Read the model definition and answer for the solid it produces. Units are mm, in the model's axes. A direction names the side the tool comes from. Coordinates: 2 decimals unless noted, no trailing zeros. Write each loop counter-clockwise with the first axis right and the second up, starting at its lowest first coordinate (ties: lowest second). Pieces come first, ordered by that corner, then holes.
(1) Find the intervals of material crossed by probe 1 along Y at (x, z) = (-76, -3); probe 2 along Z at (x, y) = (-47, -22); probe 3 along Z at (x, y) = (-68, -23.5), in increasing order.
(2) Given pin 1 (1 mm diameter, centred on x = -35, y = -8.5, fed in from +Z); pin 2 (6 mm diameter, centred on x = -29, z = -38, fed in from +Y); pin 3 (8 mm diameter, centred on x = -19, y = -14, fed in from +Z); pin 4 (4 mm diameter, centred on x = -33.5, y = -19.5, fed in from -Z), each flat-ended and moving along its own axis, determine where each tip first touches the part or whether it passes through.
(3) The mould has two halves that part along Z. Classify faces 1 (the cylindrical face through (-58.34, -3.22, 16.94)), 2 (the cylindrical face through (-85.704, -15.653, -1.885)), 3 (the flat face through (-33, 0, 1)): +Z half, -Z half, draft (parallel to the pull), parting line (faces both ways), or undercut.
(4) Section A-A on x = -27.5 is taken. Write down the section's boundary in (y, z), then the cut area to 3 significant figures.
(5) Which of the six approach directions +Z, -Z, +X, -X, +Y, -Y give full straight-line access (tool end or side, diameter ignored) to faces 4 (the flat face through (-31, -6.35, 1)), 5 (the cylindrical face through (-36.031, -3.219, -48.252))?
(6) Section D-D on x = -7.5 is taken. Write down the section's boundary in (y, z), then the cut area to 3 significant figures.
Autodesk Inventor part; units mm, degrees
ref_plane "YZ Plane" through (0, 0, 0) normal (1, 0, 0) x (0, 1, 0)
ref_plane "XZ Plane" through (0, 0, 0) normal (0, 1, 0) x (-1, 0, 0)
ref_plane "XY Plane" through (0, 0, 0) normal (0, 0, 1) x (1, 0, 0)
sketch "Sketch1" plane through (0, 0, 0) normal (0, 1, 0) x (-1, 0, 0)
  circle A0 centre (0, 0) radius 85.725
  dimension "d0" = 171.45
extrude "Extrusion1" add sketch "Sketch1" against normal blind 6.35
sketch "Sketch2" plane through (0, -6.35, 0) normal (0, -1, 0) x (1, 0, 0)
  circle A0 centre (0, 0) radius 85.725
  circle A1 centre (0, 0) radius 80.9625
  dimension "d3" = 161.925
extrude "Extrusion2" add sketch "Sketch2" along normal blind 25.4
sketch "Sketch3" plane through (0, 0, 0) normal (0, 1, 0) x (1, 0, 0)
  arc A0 (0, -85.725) -> (0, 85.725) centre (0, 0) ccw
  circle A1 centre (0, 0) radius 85.725
  line L0 (0, 85.725) -> (0, -85.725)
extrude "Extrusion3" cut sketch "Sketch3" against normal through all contours L0 A0
sketch "Sketch4" plane through (0, 0, 0) normal (0, 1, 0) x (1, 0, 0)
  circle A0 centre (0, 0) radius 63.5 construction
  line L0 (0, 0) -> (-37.3244, -51.3726) construction
  line L1 (0, -85.725) -> (0, 85.725) construction
  point P0 (-60.3921, -19.6226)
  point P1 (-60.3921, 19.6226)
  point P2 (-37.3244, 51.3726)
  point P3 (0, 63.5)
  point P4 (37.3244, 51.3726)
  point P5 (60.3921, 19.6226)
  point P6 (60.3921, -19.6226)
  point P7 (37.3244, -51.3726)
  point P8 (0, -63.5)
  dimension "d8" = 127
  dimension "d9" = 36
  dimension "d12" = 360
hole "Hole1" at (-37.3244, 0, 51.3726) at (-60.3921, 0, 19.6226) at (-60.3921, 0, -19.6226) at (-37.3244, 0, -51.3726) at (0, 0, -63.5) at (37.3244, 0, -51.3726) at (60.3921, 0, -19.6226) at (60.3921, 0, 19.6226) at (37.3244, 0, 51.3726) at (0, 0, 63.5) direction (0, -1, 0) diameter 6.7564 end through all
properties part number "CoverPlateForWaterHalf" material "PET Plastic"
Response:
1. probe 1: y = -6.35 to 0
1. probe 2: z = -71.69 to -65.92, 65.92 to 71.69
1. probe 3: z = -52.2 to -43.94, 43.94 to 52.2
2. pin 1: stops at z = 78.48
2. pin 2: stops at y = 0
2. pin 3: stops at z = 84.4
2. pin 4: stops at z = -79.73
3. face 1: undercut
3. face 2: parting line
3. face 3: draft
4. outline: (-31.75, -81.19) - (0, -81.19) - (0, 81.19) - (-31.75, 81.19) - (-31.75, 76.15) - (-6.35, 76.15) - (-6.35, -76.15) - (-31.75, -76.15) - close
4. area: 1,290 mm2
5. face 4: +X, -Y
5. face 5: +Y, -Y
6. outline: (-31.75, -85.4) - (0, -85.4) - (0, 85.4) - (-31.75, 85.4) - (-31.75, 80.61) - (-6.35, 80.61) - (-6.35, -80.61) - (-31.75, -80.61) - close
6. area: 1,330 mm2
